from build123d import *

# Parameters (mm, degrees)
BOSS_EXTRUDE1_DEPTH = 25
CHAMFER1_SIZE       = 0.4


with BuildPart() as part:
    # Sketch1 → Boss-Extrude1 (new, symmetric)
    with BuildSketch(Plane(origin=(0, 0, 0), x_dir=(0, 0, -1), z_dir=(1, 0, 0))):
        with BuildLine():
            Line((0.995546671, 1.439231331), (-0.995546671, 1.439231331))
            ThreePointArc((-0.995546671, 1.439231331), (0, -1.75), (0.995546671, 1.439231331))
        make_face()
    extrude(amount=BOSS_EXTRUDE1_DEPTH, both=True)

    # Chamfer1
    # the kernel refuses this chamfer: 0.4 mm, written as the material it takes off along each edge
    with BuildSketch(Plane(origin=(-25, 1.439231331, -2.024219866), x_dir=(0.9996219169112966, 0.02749587661058634, 0), z_dir=(0, 0, 1))) as chamfer1_piece_1:
        Polygon((CHAMFER1_SIZE * 0.999621916911, -CHAMFER1_SIZE * 0.0274958766106), (-CHAMFER1_SIZE * 0.0274958766106, -CHAMFER1_SIZE * 0.999621916911), (0, 0), align=None)
    extrude(amount=4.048439733, mode=Mode.SUBTRACT)
    with BuildSketch(Plane(origin=(-25, 0, 0), x_dir=(0, 0.9998895110785412, 0.014864912886252453), z_dir=(0, 0.014864912886252453, -0.9998895110785412))) as chamfer1_piece_2:
        Polygon((1.75, CHAMFER1_SIZE), (1.75 - CHAMFER1_SIZE, 0), (1.75, 0), align=None)
    revolve(axis=Axis((-25, 0, 0), (1, 0, 0)), revolution_arc=358.296543719, mode=Mode.SUBTRACT)
    with BuildSketch(Plane(origin=(25, 0, 0), x_dir=(0, 0.9998895110785412, 0.014864912886252453), z_dir=(0, 0.014864912886252453, -0.9998895110785412))) as chamfer1_piece_3:
        Polygon((1.75 - CHAMFER1_SIZE, 0), (1.75, -CHAMFER1_SIZE), (1.75, 0), align=None)
    revolve(axis=Axis((25, 0, 0), (1, 0, 0)), revolution_arc=358.296543719, mode=Mode.SUBTRACT)
    with BuildSketch(Plane(origin=(25, 1.439231331, -2.024219866), x_dir=(-0.9996219169112966, 0.02749587661058634, 0), z_dir=(0, 0, 1))) as chamfer1_piece_4:
        Polygon((CHAMFER1_SIZE * 0.999621916911, CHAMFER1_SIZE * 0.0274958766106), (-CHAMFER1_SIZE * 0.0274958766106, CHAMFER1_SIZE * 0.999621916911), (0, 0), align=None)
    extrude(amount=4.048439733, mode=Mode.SUBTRACT)


solid = part.part
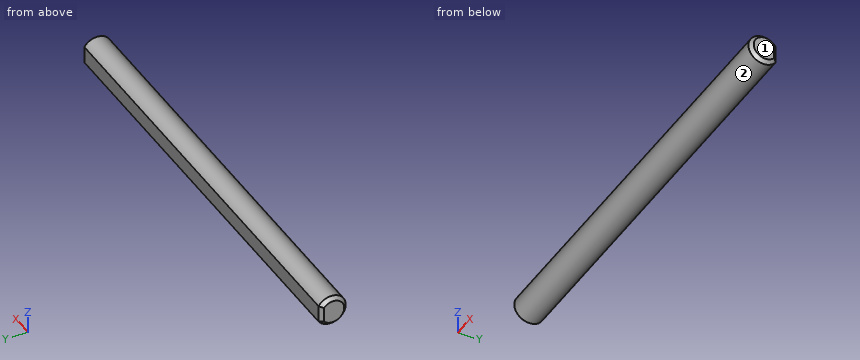
Geometry check sheet. Reference: the model listing, model coordinates, mm. Face numbers are marked on the shaded views. Give positions to 0.01 mm unless a question says otherwise; leave off trailing zeros. Write each loop counter-clockwise with the first axis right and the second up, starting at its lowest first coordinate (ties: lowest second). Pieces come first, ordered by that corner, then holes.
1) Release check for a two-part mould opening along Z. For the marked faces 1 and 2 record: released by +Z, released by -Z, zero draft, split by the parting line, or undercut.
Values follow:
face 1: zero draft
face 2: split by the parting line
2) Thickness scan on line 1 (X direction, y = 0.85, z = -1.05); line 2 (Y direction, x = 1, z = -1.1); line 3 (Y direction, x = -13, z = 1.25). Record the ranges inside material, lowest first.
Values follow:
line 1: x = -25 to 25
line 2: y = -1.36 to 1.36
line 3: y = -1.22 to 1.22
3) Cross-section at A-A (x = 9.5). Record the boundary of the cut face in (y, z).
Values follow:
outline: (1.44, -1) - (1.44, 1) arc R1.75 ccw (long way) to start
4) Go/stop test with a flat-tipped pin: pin 1 Ø1.5 at (x, y) = (-12.5, -1) entering from +Z. Record where the tip stops, or that it passes through.
Values follow:
pin 1: stops at z = 1.73
